```python
from build123d import *

# Parameters (mm, degrees)
SKETCH1_W                = 38.5
SKETCH1_H                = 38
SKETCH1_R                = 10
BOSS_EXTRUDE1_DEPTH      = 2
BOSS_EXTRUDE2_DEPTH      = 14
BOSS_EXTRUDE2_DEPTH_BACK = 2
CUT_EXTRUDE1_REACH       = 50.345
SKETCH3_W                = 10
SKETCH3_H                = 2.5
CUT_EXTRUDE2_DEPTH       = 47.384938288
CUT_EXTRUDE2_DRAFT       = 15
FILLET1_R                = 1


with BuildPart() as part:
    # Sketch1 → Boss-Extrude1 (new body)
    with BuildSketch(Plane.XY):
        Rectangle(SKETCH1_W, SKETCH1_H)
        Circle(SKETCH1_R, mode=Mode.SUBTRACT)
    extrude(amount=BOSS_EXTRUDE1_DEPTH)

    # Sketch2 → Boss-Extrude2 (add, two sides: drawn at the far end of the back side and taken through both)
    with BuildSketch(Plane.XY.offset(2).offset(-BOSS_EXTRUDE2_DEPTH_BACK)):
        Polygon((-21.25, -19), (-19.25, -19), (-19.25, 19), (19.25, 19), (19.25, -19), (21.25, -19), (21.25, 21), (-21.25, 21), align=None)
    extrude(amount=BOSS_EXTRUDE2_DEPTH + BOSS_EXTRUDE2_DEPTH_BACK)

    # Sketch3 → Cut-Extrude1 (cut, up to next)
    with BuildSketch(Plane(origin=(-19.25, 0, 0), x_dir=(0, 0, -1), z_dir=(1, 0, 0)), mode=Mode.PRIVATE) as cut_extrude1_sk1:
        with Locations((-11, 0)):
            Rectangle(SKETCH3_W, SKETCH3_H)
    cut_extrude1_tool1 = extrude(cut_extrude1_sk1.sketch, amount=-CUT_EXTRUDE1_REACH, mode=Mode.PRIVATE) & part.part
    cut_extrude1 = cut_extrude1_tool1.solids().sort_by_distance((-19.25, 0, 11))[0]
    add(cut_extrude1, mode=Mode.SUBTRACT)

    # Mirror1: Cut-Extrude1 across plane
    add(cut_extrude1.mirror(Plane(origin=(0, 0, 0), x_dir=(0, 0, 1), z_dir=(1, 0, 0))), mode=Mode.SUBTRACT)


with BuildPart() as cut_extrude2_tool:
    # Sketch5 → Cut-Extrude2 (with draft: the straight prism first)
    with BuildSketch(Plane.XZ.offset(-19)):
        with BuildLine():
            ThreePointArc((-5, 13.591034656), (-7.5, 11.091034656), (-5, 8.591034656))
            Line((-5, 8.591034656), (5, 8.591034656))
            ThreePointArc((5, 8.591034656), (7.5, 11.091034656), (5, 13.591034656))
            Line((5, 13.591034656), (-5, 13.591034656))
        make_face()
    extrude(amount=-CUT_EXTRUDE2_DEPTH)
    # Cut-Extrude2: the draft: its side faces are tilted about the plane it starts from
    cut_extrude2_sides = [cut_extrude2_tool.faces().sort_by_distance(p)[0] for p in [
        (-7.5, 42.692469144, 11.091034656),
        (0, 42.692469144, 8.591034656),
        (7.5, 42.692469144, 11.091034656),
        (0, 42.692469144, 13.591034656),
    ]]
    draft(cut_extrude2_sides, Plane.XZ.offset(-19), CUT_EXTRUDE2_DRAFT)


with BuildPart() as part_1:
    add(part.part)

    # Cut-Extrude2: cut by cut_extrude2_tool
    add(cut_extrude2_tool.part, mode=Mode.SUBTRACT)

    # Fillet1
    fillet1_edges = [part_1.edges().sort_by_distance(p)[0] for p in [
        (-7.5, 19, 11.091034656),
        (0, 19, 8.591034656),
        (7.5, 19, 11.091034656),
        (0, 19, 13.591034656),
    ]]
    fillet(fillet1_edges, radius=FILLET1_R)


solid = part_1.part
```
Geometry check sheet. Reference: the model listing, model coordinates, mm. A direction names the side the tool comes from. Give positions to 0.01 mm unless a question says otherwise; leave off trailing zeros. Order: outer loops, then holes, each group sorted by start corner. A loop starts at its lowest first (then second) coordinate and runs counter-clockwise, first axis right, second up. Notation, with made-up numbers: (69, 56) - (74, 56) arc R18 ccw to (74, 69) - close; hole circle Ø4 at (13.25, 34.25). An arc over 180 degrees is marked (long way). Answer in a Markdown table with one row per item. Add a question column.
Q1. Material ranges on probe 1 along X at (y, z) = (15, 2.25); probe 2 along Y at (x, z) = (0, 1); probe 3 along Z at (x, y) = (16.5, -3), recorded low to high. Write a range as from..to.
Q2. Cross-section at A-A, the plane x = 0. Enter the section's corners in (y, z), then the cut area to 3 significant figures.
Q3. Gauge pin test, flat ends, axial feed: pin 1 (11.5 mm diameter, centred on x = -2.5, y = -5.5, fed in from +Z); pin 2 (1 mm diameter, centred on x = 20, y = 0.5, fed in from +Z); pin 3 (4 mm diameter, centred on x = -0.5, z = 5.5, fed in from -Y). Record the tip position at first contact, or that the pin passes through.
Q4. Cross-section at D-D, the plane x = 18. Enter the section's corners in (y, z).
Q5. Cross-section at B-B, the plane y = 0. Enter the section's corners in (x, z).
Q6. Mould release check, pull along Z, two halves, no side actions. Record for faces 1 (the flat face through (20, 1.25, 11)), 2 (the conical face through (-7.9, 20.5, 11.2)), 3 (the flat face through (-9, 9, 2)): pulls with the +Z half, pulls with the -Z half, needs draft (parallel to the pull), parting line crosses it, or undercut.
Q7. Tool access check on faces 4 (the conical face through (7.9, 20.5, 11)), 5 (the flat face through (20, -10, 16)), 6 (the flat face through (20, -1.25, 11)), 7 (the flat face through (0, 19, 6)), 8 (the flat face through (0, -19, 1)). Record the directions out of +Z, -Z, +X, -X, +Y, -Y that give a thin tool (end or side, any length) a straight path to the whole face; none if there is none.
Q8. Cross-section at C-C, the plane y = 15. Enter the section's corners in (x, z), then the cut area to 3 significant figures.
Check values:
| question | item | result |
|---|---|---|
| 1 | probe 1 | x = -21.25..-19.25, 19.25..21.25 |
| 1 | probe 2 | y = -19..-10, 10..21 |
| 1 | probe 3 | z = 0..2 |
| 2 | outline | (-19, 0) - (-10, 0) - (-10, 2) - (-19, 2) - close; (10, 0) - (21, 0) - (21, 8.06) - (20.26, 8.25) arc R1 ccw to (19, 7.29) - (19, 2) - (10, 2) - close; (19, 14.89) arc R1 ccw to (20.26, 13.93) - (21, 14.13) - (21, 16) - (19, 16) - close |
| 2 | area | 56.2 mm^2 |
| 3 | pin 1 | stops at z = 2 |
| 3 | pin 2 | stops at z = 6 |
| 3 | pin 3 | stops at y = 19 |
| 4 | outline | (-19, 0) - (21, 0) - (21, 16) - (19, 16) - (19, 2) - (-19, 2) - close |
| 5 | outline | (-21.25, 0) - (-10, 0) - (-10, 2) - (-19.25, 2) - (-19.25, 6) - (-21.25, 6) - close; (10, 0) - (21.25, 0) - (21.25, 6) - (19.25, 6) - (19.25, 2) - (10, 2) - close |
| 6 | face 1 | needs draft |
| 6 | face 2 | undercut |
| 6 | face 3 | pulls with the +Z half |
| 7 | face 4 | +Y |
| 7 | face 5 | +Z, +X, -X, +Y, -Y |
| 7 | face 6 | +Z, +X, -X |
| 7 | face 7 | +Z, -Y |
| 7 | face 8 | +Z, -Z, +X, -X, -Y |
| 8 | outline | (-21.25, 0) - (21.25, 0) - (21.25, 16) - (19.25, 16) - (19.25, 2) - (-19.25, 2) - (-19.25, 16) - (-21.25, 16) - close |
| 8 | area | 141 mm^2 |
